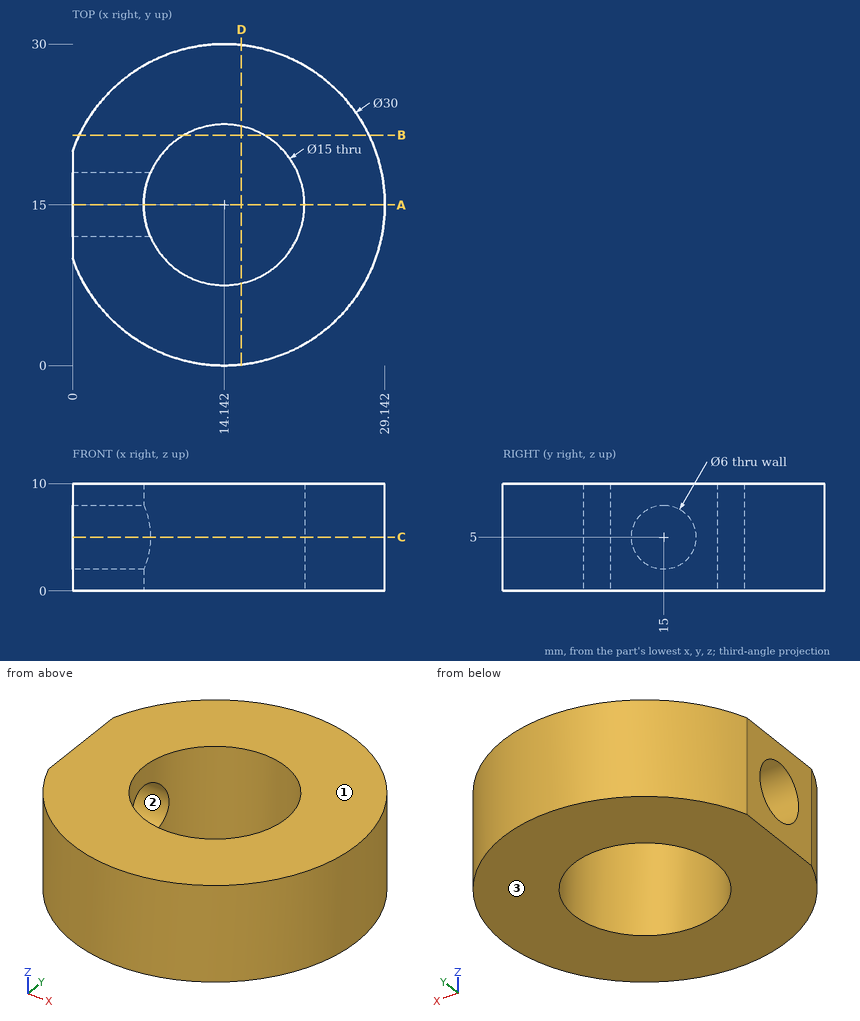
Job drawing, mm, ordinate dimensions from the low corner. One solid piece. Give positions to 0.01 mm unless a question says otherwise; leave off trailing zeros. Loops run counter-clockwise (first coordinate to the right, second up) from the corner with the lowest first, then second, coordinate; pieces in that order, holes last.
Item 1: Drill centre lines: line 1 (Z direction, x = 3.5, y = 15); line 2 (Y direction, x = 14, z = 9.5); line 3 (Y direction, x = 9.75, z = 2). Where is each one in solid material? Low to high.
Answers follow:
line 1: z = 0 to 2, 8 to 10
line 2: y = 0 to 7.5, 22.5 to 30
line 3: y = 0.66 to 8.92, 21.08 to 29.34
Item 2: Slice it at D-D, the plane x = 15.75. List the corners of the cut face in (y, z).
Answers follow:
outline: (0.09, 0) - (7.67, 0) - (7.67, 10) - (0.09, 10) - close; (22.33, 0) - (29.91, 0) - (29.91, 10) - (22.33, 10) - close
Item 3: Slice it at B-B, the plane y = 21.5. List the corners of the cut face in (x, z).
Answers follow:
outline: (0.62, 0) - (10.4, 0) - (10.4, 10) - (0.62, 10) - close; (17.88, 0) - (27.66, 0) - (27.66, 10) - (17.88, 10) - close
Item 4: Slice it at C-C, the plane z = 5. List the corners of the cut face in (x, y), and give its area (3 significant figures).
Answers follow:
outline: (0, 10) arc R15 ccw (long way) to (0, 20) - (0, 18) - (7.27, 18) arc R7.5 cw (long way) to (7.27, 12) - (0, 12) - close
area: 483 mm2
Item 5: Flat gauge pins, fed straight in: pin 1 (4 mm diameter, centred on x = 25, z = 4, fed in from -Y) (1 decimal); pin 2 (1 mm diameter, centred on y = 8, z = 6, fed in from -X); pin 3 (1 mm diameter, centred on y = 5.5, z = 7, fed in from -X). Where does each tip first touch, or does it go through?
Answers follow:
pin 1: stops at y = 2.9
pin 2: stops at x = 0.62
pin 3: stops at x = 2.14
Item 6: Pull direction Z, two halves, no side cores. Call the marked faces 1, 2 and 3: released by +Z, released by -Z, zero draft, split by the parting line, or undercut.
Answers follow:
face 1: released by +Z
face 2: undercut
face 3: released by -Z
Item 7: Slice it at A-A, the plane y = 15. List the corners of the cut face in (x, z), and give its area (3 significant figures).
Answers follow:
outline: (0, 0) - (6.64, 0) - (6.64, 2) - (0, 2) - close; (0, 8) - (6.64, 8) - (6.64, 10) - (0, 10) - close; (21.64, 0) - (29.14, 0) - (29.14, 10) - (21.64, 10) - close
area: 102 mm2
